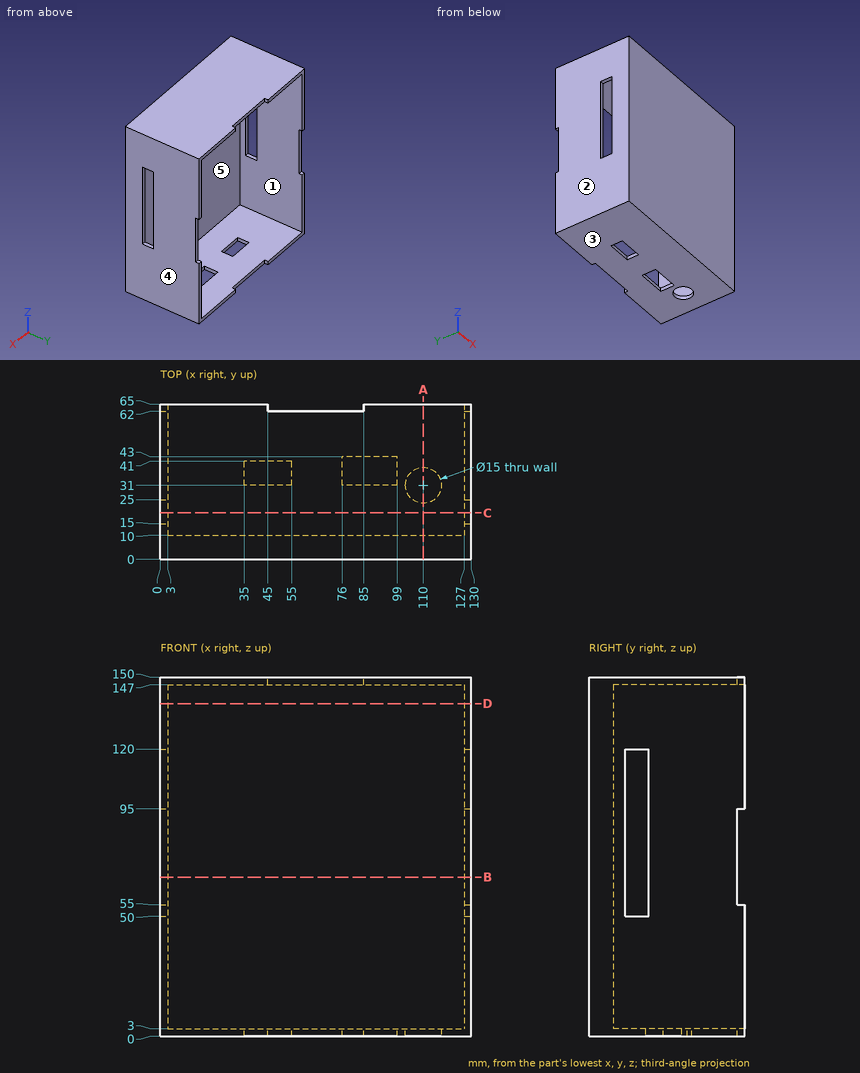
Design review of the part shown in the three views and the two pictorial views. Dimensions are in mm from the part's minimum x, y and z. A direction names the side the tool comes from. Give positions to 0.01 mm unless a question says otherwise; leave off trailing zeros. Loops run counter-clockwise (first coordinate to the right, second up) from the corner with the lowest first, then second, coordinate; pieces in that order, holes last. Notation, with made-up numbers: (11, 9) -> (44, 9) arc R19 cw to (44, 38) -> close; hole circle Ø2 at (74, -20). An arc over 180 degrees is marked (long way). One line per question, with ' | ' between items.
1) We need section A-A (x = 110). Write out the cut boundary in (y, z), plus the area to 4 significant figures.
Resolved:
outline: (0, 0) -> (23.5, 0) -> (23.5, 3) -> (10, 3) -> (10, 147) -> (65, 147) -> (65, 150) -> (0, 150) -> close; (38.5, 0) -> (65, 0) -> (65, 3) -> (38.5, 3) -> close | area: 1,785 mm2
2) For the marked faces 4 and 5, list the 3-axis set-ups (+Z, -Z, +X, -X, +Y, -Y) from which the entire face can be reached by the end or side of a thin tool; tool diameter is ignored.
Resolved:
face 4: +Z, -Z, +X, +Y, -Y | face 5: +Y
3) Insertion check: pin 1 Ø2.5 at (x, z) = (67, 148.5) entering from +Y; pin 2 Ø1.5 at (x, y) = (1, 18.5) entering from -Z; pin 3 Ø2 at (x, z) = (63, 132) entering from +Y; pin 4 Ø12 at (x, y) = (110, 31) entering from -Z. Each pin has a flat end and moves straight along its axis. Give the tip position at first contact, or say it passes through.
Resolved:
pin 1: stops at y = 62 | pin 2: stops at z = 0 | pin 3: stops at y = 10 | pin 4: stops at z = 147
4) We need section D-D (z = 139). Write out the cut boundary in (x, y).
Resolved:
outline: (0, 0) -> (130, 0) -> (130, 65) -> (127, 65) -> (127, 10) -> (3, 10) -> (3, 65) -> (0, 65) -> close
5) We need section C-C (y = 19.5). Write out the cut boundary in (x, z), plus the area to 3 significant figures.
Resolved:
outline: (0, 0) -> (130, 0) -> (130, 50) -> (127, 50) -> (127, 3) -> (3, 3) -> (3, 50) -> (0, 50) -> close; (0, 120) -> (3, 120) -> (3, 147) -> (127, 147) -> (127, 120) -> (130, 120) -> (130, 150) -> (0, 150) -> close | area: 1,220 mm2
6) We need section B-B (z = 66.5). Write out the cut boundary in (x, y).
Resolved:
outline: (0, 0) -> (130, 0) -> (130, 15) -> (127, 15) -> (127, 10) -> (3, 10) -> (3, 15) -> (0, 15) -> close; (0, 25) -> (3, 25) -> (3, 62) -> (0, 62) -> close; (127, 25) -> (130, 25) -> (130, 62) -> (127, 62) -> close
7) To check wall thickness, follow probe 1 along Z at (x, y) = (63.5, 42.5); probe 2 along Y at (x, z) = (110, 0.7); probe 3 along X at (y, z) = (49.5, 141.5). State the ranges of each line that lie inside material, in increasing order.
Resolved:
probe 1: z = 0 to 3, 147 to 150 | probe 2: y = 0 to 23.5, 38.5 to 65 | probe 3: x = 0 to 3, 127 to 130
8) The part is to be moulded in two halves that separate along Z. For the marked faces 1, 2 and 3, say which applies: +Z half, -Z half, draft (parallel to the pull), parting line (faces both ways), or undercut.
Resolved:
face 1: undercut | face 2: draft | face 3: -Z half
